Could you check a few things on this drawing? It's one solid part, dimensions in mm from its lowest x, y, z. Give positions to 0.01 mm unless a question says otherwise; leave off trailing zeros. Loops run counter-clockwise (first coordinate to the right, second up) from the corner with the lowest first, then second, coordinate; pieces in that order, holes last. Notation, with made-up numbers: (-10, 25) - (9, 25) arc R27 cw to (9, 49) - close; hole circle Ø3 at (-35, 38). An arc over 180 degrees is marked (long way). Write item = value, one per line.
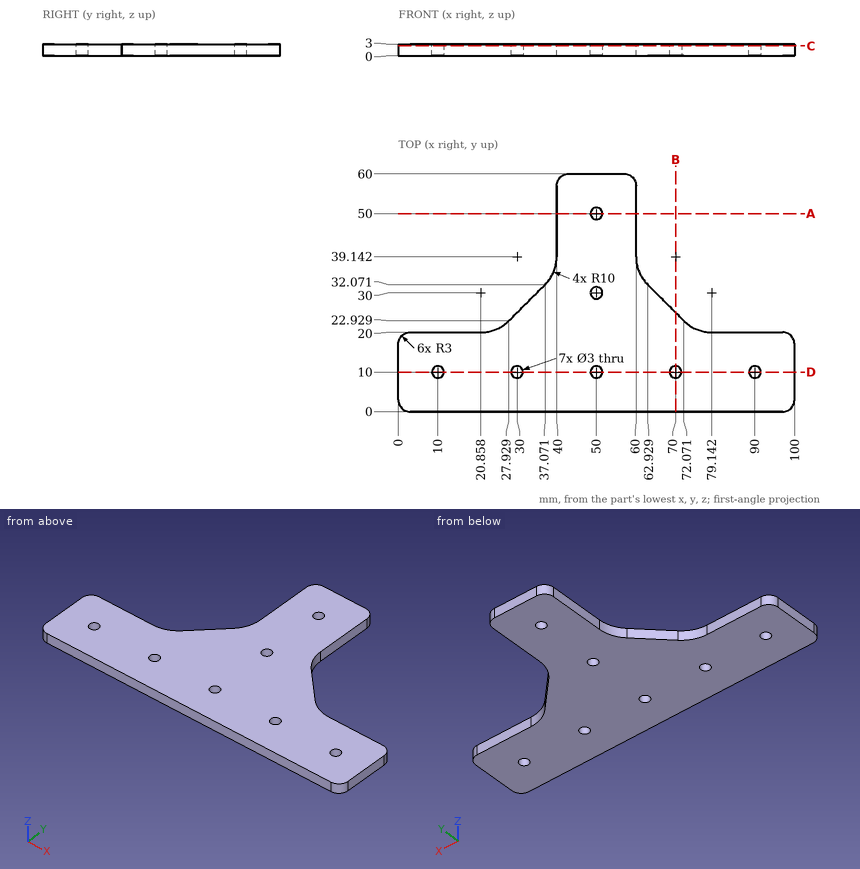
Q1. Imagine slicing it at D-D, the plane y = 10. Write out the boundary of the cut face in (x, z).
Output:
outline = (0, 0) - (8.5, 0) - (8.5, 3) - (0, 3) - close; (11.5, 0) - (28.5, 0) - (28.5, 3) - (11.5, 3) - close; (31.5, 0) - (48.5, 0) - (48.5, 3) - (31.5, 3) - close; (51.5, 0) - (68.5, 0) - (68.5, 3) - (51.5, 3) - close; (71.5, 0) - (88.5, 0) - (88.5, 3) - (71.5, 3) - close; (91.5, 0) - (100, 0) - (100, 3) - (91.5, 3) - close
Q2. For pin 1 (1 mm diameter, centred on y = 31.5, z = 1.5, fed in from -X); pin 2 (1.5 mm diameter, centred on y = 37.5, z = 2.5, fed in from +X), each with a flat end and sliding along its axis, tell me the tip position at first contact or that it passes through.
Output:
pin_1 = 36
pin_2 = 60.29
Q3. Imagine slicing it at C-C, the plane z = 2.5. Write out the boundary of the cut face in (x, y), then the cut area to 3 significant figures.
Output:
outline = (0, 3) arc R3 ccw to (3, 0) - (97, 0) arc R3 ccw to (100, 3) - (100, 17) arc R3 ccw to (97, 20) - (79.14, 20) arc R10 cw to (72.07, 22.93) - (62.93, 32.07) arc R10 cw to (60, 39.14) - (60, 57) arc R3 ccw to (57, 60) - (43, 60) arc R3 ccw to (40, 57) - (40, 39.14) arc R10 cw to (37.07, 32.07) - (27.93, 22.93) arc R10 cw to (20.86, 20) - (3, 20) arc R3 ccw to (0, 17) - close; hole circle Ø3 at (10, 10); hole circle Ø3 at (30, 10); hole circle Ø3 at (50, 10); hole circle Ø3 at (50, 30); hole circle Ø3 at (50, 50); hole circle Ø3 at (70, 10); hole circle Ø3 at (90, 10)
area = 2,970 mm2
Q4. Imagine slicing it at A-A, the plane y = 50. Write out the boundary of the cut face in (x, z).
Output:
outline = (40, 0) - (48.5, 0) - (48.5, 3) - (40, 3) - close; (51.5, 0) - (60, 0) - (60, 3) - (51.5, 3) - close
Q5. I need wall thicknesses on L1, parallel to Y at x = 50, z = 1.4; L2, parallel to Y at x = 10, z = 1.25; L3, parallel to X at y = 56, z = 2.15. Which ranges of each line are inside material? Lowest first, please.
Output:
L1 = 0 to 8.5, 11.5 to 28.5, 31.5 to 48.5, 51.5 to 60
L2 = 0 to 8.5, 11.5 to 20
L3 = 40 to 60
Q6. Imagine slicing it at B-B, the plane x = 70. Write out the boundary of the cut face in (y, z).
Output:
outline = (0, 0) - (8.5, 0) - (8.5, 3) - (0, 3) - close; (11.5, 0) - (25, 0) - (25, 3) - (11.5, 3) - close
